Input: part model. Units: mm. Frame: model coordinates. A direction names the side the tool comes from. Coordinates: 2 decimals unless noted, no trailing zeros. Loops run counter-clockwise (first coordinate to the right, second up) from the corner with the lowest first, then second, coordinate; pieces in that order, holes last.
```python
from build123d import *

# Parameters (mm, degrees)
CYLINDER001_R               = 4
CYLINDER001_DEPTH           = 13
CYLINDER001_PLACEMENT_ANGLE = 2
ARRAY_COUNT                 = 8
CYLINDER_R                  = 20
CYLINDER_DEPTH              = 15
CHAMFER_SIZE                = 1


with BuildPart() as array:
    # Cylinder001 → Cylinder001 (new body)
    with BuildSketch(Plane.XY):
        Circle(CYLINDER001_R)
    extrude(amount=CYLINDER001_DEPTH)


with BuildPart() as array_1:
    # Cylinder001 placement: moved
    add(array.part.moved(Location((20, 0, 5))).rotate(Axis((20, 0, 5), (0, 0, -1)), CYLINDER001_PLACEMENT_ANGLE))

    # Array: Array ×8 about axis
    array_axis = Axis((0, 0, 0), (0, 0, 1))


with BuildPart() as array_2:
    add(array_1.part)
    for i in range(1, ARRAY_COUNT):
        add(array_1.part.rotate(array_axis, i * 360 / ARRAY_COUNT))


with BuildPart() as chamfer_body:
    # Cylinder → Cylinder (new body)
    with BuildSketch(Plane.XY):
        Circle(CYLINDER_R)
    extrude(amount=CYLINDER_DEPTH)

    # Cut: cut Array
    add(array_2.part, mode=Mode.SUBTRACT)

    # Chamfer
    chamfer_edges = [chamfer_body.edges().sort_by_distance(p)[0] for p in [
        (18.477591, 7.653669, 15),
        (7.653669, 18.477591, 15),
        (-7.653669, 18.477591, 15),
        (-18.477591, 7.653669, 15),
        (-18.477591, -7.653669, 15),
        (-7.653669, -18.477591, 15),
        (7.653669, -18.477591, 15),
        (18.477591, -7.653669, 15),
        (16, 0, 15),
        (11.313708, -11.313708, 15),
        (0, -16, 15),
        (-11.313708, -11.313708, 15),
        (-16, 0, 15),
        (-11.313708, 11.313708, 15),
        (0, 16, 15),
        (11.313708, 11.313708, 15),
    ]]
    chamfer(chamfer_edges, length=CHAMFER_SIZE)


solid = chamfer_body.part
```
Item 1: Line query: L1, parallel to X at y = 10.5, z = 14.25; L2, parallel to Y at x = -4, z = 2; L3, parallel to Y at x = 17.5, z = 10.75. Output: solid intervals per line, ascending.
Result:
L1: x = -16.73 to -16.33, -11.95 to 11.95, 16.33 to 16.73
L2: y = -19.6 to 19.6
L3: y = -9.68 to -3.12, 3.12 to 9.68
Item 2: Mould query, pull axis Y, two halves, no side actions, for faces 1 (the face through (11.37, -11.26, 9.44)), 2 (the face through (-7.411, 18.029, 14.507)), 3 (the face through (0, 18, 5)). Classes: +Y half, -Y half, draft (parallel to the pull), parting line (faces both ways), or undercut.
Result:
face 1: undercut
face 2: +Y half
face 3: draft
Item 3: Section query A-A (x = 0). Output: boundary loops of the cut face in (y, z), then the cut area to 3 significant figures.
Result:
outline: (-20, 0) - (20, 0) - (20, 5) - (16, 5) - (16, 14) - (15, 15) - (-15, 15) - (-16, 14) - (-16, 5) - (-20, 5) - close
area: 519 mm2
Item 4: Reachability of faces 4 (the face through (0, 16, 9)), 5 (the face through (0, -16, 9)), 6 (the face through (-16, 0, 9)), 7 (the face through (18, 0, 5)), 8 (the face through (13, 13, 5)) from +Z, -Z, +X, -X, +Y, -Y: full face, straight path, thin tool, end or side. Return the list, or none.
Result:
face 4: +Z, +Y
face 5: +Z, -Y
face 6: +Z, -X
face 7: +Z, +X
face 8: +Z
Item 5: Contact query for flat-ended pins moving along their axis: P1, Ø2, axis at x = 15, y = -12, coming from the +Z side; P2, Ø2, axis at y = 6, z = 11.5, coming from the -X side; P3, Ø1, axis at y = 14, z = 11.5, coming from the -X side. Output: stop coordinate, or through.
Result:
P1: stops at z = 5
P2: stops at x = -19.36
P3: stops at x = -10.19
Item 6: Section query B-B (z = 10.25). Output: boundary loops of the cut face in (x, y).
Result:
outline: (-19.6, -3.98) arc R20 ccw to (-16.67, -11.05) arc R4 cw to (-11.05, -16.67) arc R20 ccw to (-3.98, -19.6) arc R4 cw to (3.98, -19.6) arc R20 ccw to (11.05, -16.67) arc R4 cw to (16.67, -11.05) arc R20 ccw to (19.6, -3.98) arc R4 cw to (19.6, 3.98) arc R20 ccw to (16.67, 11.05) arc R4 cw to (11.05, 16.67) arc R20 ccw to (3.98, 19.6) arc R4 cw to (-3.98, 19.6) arc R20 ccw to (-11.05, 16.67) arc R4 cw to (-16.67, 11.05) arc R20 ccw to (-19.6, 3.98) arc R4 cw to start
